from build123d import *

# Parameters (mm, degrees)
BASENUT_DEPTH   = 5.3
SKETCH3_R       = 1.7
HOLE_DEPTH      = 6.3
ENDCHAMFER_SIZE = 0.485714286


with BuildPart() as part:
    # Sketch1 → BaseNut (new body)
    with BuildSketch(Plane.XY):
        Polygon((2.309401077, -4), (4.618802154, 0), (2.309401077, 4), (-2.309401077, 4), (-4.618802154, 0), (-2.309401077, -4), align=None)
    extrude(amount=-BASENUT_DEPTH)

    # Sketch2 → Double-Chamfer (revolve, cut)
    with BuildSketch(Plane(origin=(0.481162538, 0, -5.099964691), x_dir=(0, 0, -1), z_dir=(0, -1, 0))):
        Polygon((-0.115823776, 4.137639616), (0.200035309, 4.137639616), (0.200035309, 2.958837462), align=None)
        Polygon((-5.099964691, 4.137639616), (-3.319964691, 4.137639616), (-5.099964691, 3.518837462), align=None)
    revolve(axis=Axis((0, 0, -4.462865094), (0, 0, 1)), mode=Mode.SUBTRACT)

    # Sketch3 → Hole (cut, through all)
    with BuildSketch(Plane.XY):
        Circle(SKETCH3_R)
    extrude(amount=-HOLE_DEPTH, mode=Mode.SUBTRACT)

    # EndChamfer
    endchamfer_edges = [part.edges().sort_by_distance(p)[0] for p in [
        (-1.7, 0, -5.3),
    ]]
    chamfer(endchamfer_edges, length=ENDCHAMFER_SIZE)


solid = part.part
Source: CAD feature listing. Evaluate the final solid. Frame: model axes, mm. Give positions to 0.01 mm unless a question says otherwise; leave off trailing zeros. Order: outer loops, then holes, each group sorted by start corner. A loop starts at its lowest first (then second) coordinate and runs counter-clockwise, first axis right, second up. Notation, with made-up numbers: (45, 56.25) -> (74, 56.25) arc R17 ccw to (74, 78.25) -> close; hole circle Ø1 at (-26.5, 53). An arc over 180 degrees is marked (long way). Use a Markdown table: item, result.
1) Mould query, pull axis X, two halves, no side actions, for faces 1 (the cylindrical face through (-0.37, -1.66, -2.37)), 2 (the conical face through (-2.083, -3.587, -0.424)), 3 (the conical face through (2.083, 3.587, -0.424)), 4 (the flat face through (0, -4, -3)). Classes: +X half, -X half, draft (parallel to the pull), parting line (faces both ways), or undercut.
Answer list:
| item | result |
|---|---|
| face 1 | undercut |
| face 2 | -X half |
| face 3 | +X half |
| face 4 | draft |
2) Section query A-A, the plane z = -1.9. Return the cut outline in (x, y), then the cut area to 3 significant figures.
Answer list:
| item | result |
|---|---|
| outline | (-4.62, 0) -> (-2.31, -4) -> (2.31, -4) -> (4.62, 0) -> (2.31, 4) -> (-2.31, 4) -> close; hole circle Ø3.4 at (0, 0) |
| area | 46.3 mm² |
3) Ray query, line 1 along Y through (x, z) = (0, -2.4); line 2 along X through (y, z) = (-0.5, -4.5); line 3 along X through (y, z) = (1, -2.3). Return the intervals inside material, ascending. Write a range as [from, to].
Answer list:
| item | result |
|---|---|
| line 1 | [-4, -1.7], [1.7, 4] |
| line 2 | [-4.33, -1.62], [1.62, 4.33] |
| line 3 | [-4.04, -1.37], [1.37, 4.04] |
